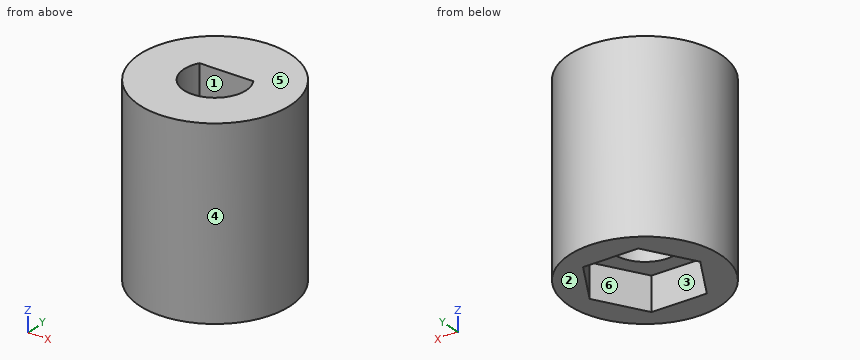
```python
from build123d import *

# Parameters (mm, degrees)
SKETCH1_R           = 4.5
BOSS_EXTRUDE1_DEPTH = 11
CUT_EXTRUDE3_DEPTH  = 2
CUT_EXTRUDE4_DEPTH  = 12


with BuildPart() as part:
    # Sketch1 → Boss-Extrude1 (new body)
    with BuildSketch(Plane.XY):
        with Locations((0, 9.145577701)):
            Circle(SKETCH1_R)
    extrude(amount=BOSS_EXTRUDE1_DEPTH)

    # Sketch6 → Cut-Extrude3 (cut)
    with BuildSketch(Plane(origin=(0, 0, 0), x_dir=(-1, 0, 0), z_dir=(0, 0, -1))):
        Polygon((3.290896534, 9.145577701), (1.645448267, 11.995577701), (-1.645448267, 11.995577701), (-3.290896534, 9.145577701), (-1.645448267, 6.295577701), (1.645448267, 6.295577701), align=None)
    extrude(amount=-CUT_EXTRUDE3_DEPTH, mode=Mode.SUBTRACT)

    # Sketch7 → Cut-Extrude4 (cut, through all)
    with BuildSketch(Plane(origin=(0, 0, 0), x_dir=(-1, 0, 0), z_dir=(0, 0, -1))):
        with BuildLine():
            Line((1.6, 10.095577701), (-1.6, 10.095577701))
            ThreePointArc((-1.6, 10.095577701), (0, 7.284798295), (1.6, 10.095577701))
        make_face()
    extrude(amount=-CUT_EXTRUDE4_DEPTH, mode=Mode.SUBTRACT)


solid = part.part
```
Can you work these out from the model? Positions are in its coordinate system, mm. Face numbers are marked on the shaded views. A direction names the side the tool comes from. Round coordinates to 2 decimals unless told otherwise and drop trailing zeros. Loops run counter-clockwise (first coordinate to the right, second up) from the corner with the lowest first, then second, coordinate; pieces in that order, holes last. Notation, with made-up numbers: M 24.5,21.25 L 77.5,21.25 A11 ccw 77.5,38.25 Z; hole C 28,24 d4. An arc over 180 degrees is marked long. Answer as a JSON object with one key per item and string values. Group by question number.
Q1. Imagine slicing it at C-C, the plane y = 9. Please give me the cut outline in (x, z), then the cut area to 3 significant figures.
Q2. Imagine slicing it at B-B, the plane z = 1.75. Please give me the cut outline in (x, y).
Q3. Please list where these lines run through material, in increasing order: L1, parallel to Y at x = 0, z = 6; L2, parallel to X at y = 8.25, z = 10.25; L3, parallel to Z at x = 0.75, y = 6.75.
Q4. We'd pull the mould along Y, two halves only. Please class the marked faces 4, 5 and 6: +Y half, -Y half, draft (parallel to the pull), parting line (faces both ways), or undercut.
Q5. On a 3-axis mill with a long thin cutter (end or side, diameter ignored), from which of +Z, -Z, +X, -X, +Y, -Y can I reach the whole of each face in a straight line? I mean the marked faces 1, 2 and 3. Say none if no direction works.
Q6. Will these pins go through, and if not, where does the flat tip stop? pin 1 (2 mm diameter, centred on x = 0, y = 9.15, fed in from -Z); pin 2 (1.5 mm diameter, centred on y = 12.5, z = 4, fed in from +X); pin 3 (4 mm diameter, centred on x = -3, z = 6, fed in from +Y).
Q7. Imagine slicing it at D-D, the plane x = -2.75. Please give me the cut outline in (y, z), then the cut area to 3 significant figures.
Q8. Imagine slicing it at A-A, the plane x = 0. Please give me the cut outline in (y, z), then the cut area to 3 significant figures.
Findings:
{
 "1": {"outline": "M -4.5,0 L -3.21,0 L -3.21,2 L -1.86,2 L -1.86,11 L -4.5,11 Z; M 1.86,2 L 3.21,2 L 3.21,0 L 4.5,0 L 4.5,11 L 1.86,11 Z", "area": "52.7 mm2"},
 "2": {"outline": "C 0,9.15 d9; hole M -3.29,9.15 L -1.65,6.3 L 1.65,6.3 L 3.29,9.15 L 1.65,12 L -1.65,12 Z"},
 "3": {"L1": "y = 4.65 to 7.28, 10.1 to 13.65", "L2": "x = -4.41 to -1.63, 1.63 to 4.41", "L3": "z = 2 to 11"},
 "4": {"face 4": "parting line", "face 5": "draft", "face 6": "undercut"},
 "5": {"face 1": "+Z, -Z", "face 2": "-Z, +X, -X, +Y, -Y", "face 3": "-Z"},
 "6": {"pin 1": "stops at z = 2", "pin 2": "stops at x = 3.67", "pin 3": "stops at y = 13.53"},
 "7": {"outline": "M 5.58,0 L 8.21,0 L 8.21,2 L 10.08,2 L 10.08,0 L 12.71,0 L 12.71,11 L 5.58,11 Z", "area": "74.6 mm2"},
 "8": {"outline": "M 4.65,0 L 6.3,0 L 6.3,2 L 7.28,2 L 7.28,11 L 4.65,11 Z; M 10.1,2 L 12,2 L 12,0 L 13.65,0 L 13.65,11 L 10.1,11 Z", "area": "62.3 mm2"}
}
